CAD build for the part. Positions are in the model's coordinates, mm. Coordinates: 2 decimals unless noted, no trailing zeros. Loops run counter-clockwise (first coordinate to the right, second up) from the corner with the lowest first, then second, coordinate; pieces in that order, holes last. Notation, with made-up numbers: (1, -5) - (30, -5) arc R26 cw to (30, 12) - close; hole circle Ø6 at (46.5, 52.25). An arc over 180 degrees is marked (long way). Put each result on its own line as item: value.
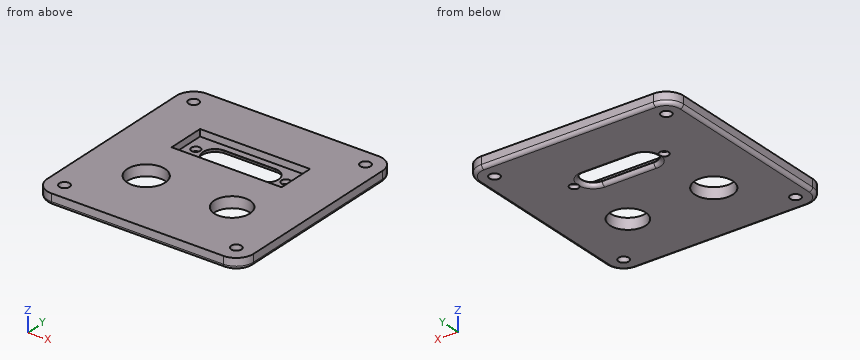
```python
from build123d import *

# Parameters (mm, degrees)
F0_W         = 76.2
F0_H         = 76.2
F0_R         = 1.905
F0_R_2       = 6.985
F0_R_3       = 6.604
F0_R_4       = 1.651
F1_DEPTH     = 1.524
F2_W         = 76.2
F2_H         = 76.2
F2_R         = 1.905
F2_W_2       = 40.64
F2_H_2       = 13.97
F3_DEPTH     = 2.54
F4_R         = 6.35
F5_T1_DEPTH  = 19.05
F5_T3_DEPTH  = 63.5
F5_T5_DEPTH  = 63.5
F5_T8_ANGLE  = 90
F5_T10_ANGLE = 90
F5_T12_ANGLE = 90
F5_T14_ANGLE = 90
F5_T16_ANGLE = 180
F5_T18_ANGLE = 180
F6_DEPTH     = 2.54


# Not quite as in the source:
# - a fillet or chamfer that OpenCascade refuses, or shapes differently, is made with other operations: its cross-section is extruded or revolved along the edge and cut away or added
# - a feature names something its author has since deleted; it is built from what else it names


with BuildPart() as f1:
    # F0 (on Top) → F1 (new body)
    with BuildSketch(Plane.XY):
        with Locations((0, -12.7)):
            Rectangle(F0_W, F0_H)
        with Locations((-31.75, -44.45)):
            Circle(F0_R, mode=Mode.SUBTRACT)
        with Locations((-15.875, -25.4)):
            Circle(F0_R_2, mode=Mode.SUBTRACT)
        with Locations((31.75, -44.45)):
            Circle(F0_R, mode=Mode.SUBTRACT)
        with Locations((15.875, -25.4)):
            Circle(F0_R_3, mode=Mode.SUBTRACT)
        with Locations((-16.637, 0)):
            Circle(F0_R_4, mode=Mode.SUBTRACT)
        with Locations((-31.75, 19.05)):
            Circle(F0_R, mode=Mode.SUBTRACT)
        with BuildLine():
            ThreePointArc((-9.525, -4.445), (-13.97, 0), (-9.525, 4.445))
            Line((-9.525, 4.445), (9.525, 4.445))
            ThreePointArc((9.525, 4.445), (13.97, 0), (9.525, -4.445))
            Line((9.525, -4.445), (-9.525, -4.445))
        make_face(mode=Mode.SUBTRACT)
        with Locations((16.637, 0)):
            Circle(F0_R_4, mode=Mode.SUBTRACT)
        with Locations((31.75, 19.05)):
            Circle(F0_R, mode=Mode.SUBTRACT)
    extrude(amount=F1_DEPTH)

    # F2 (on face) → F3 (join)
    with BuildSketch(Plane.XY.offset(1.524)):
        with Locations((0, -12.7)):
            Rectangle(F2_W, F2_H)
        with Locations((-31.75, -44.45)):
            Circle(F2_R, mode=Mode.SUBTRACT)
        with Locations((31.75, -44.45)):
            Circle(F2_R, mode=Mode.SUBTRACT)
        with Locations((-31.75, 19.05)):
            Circle(F2_R, mode=Mode.SUBTRACT)
        Rectangle(F2_W_2, F2_H_2, mode=Mode.SUBTRACT)
        with Locations((31.75, 19.05)):
            Circle(F2_R, mode=Mode.SUBTRACT)
    extrude(amount=F3_DEPTH)

    # F4
    f4_edges = [f1.edges().sort_by_distance(p)[0] for p in [
        (-38.1, -50.8, 2.032),
        (38.1, -50.8, 2.032),
        (-38.1, 25.4, 2.032),
        (38.1, 25.4, 2.032),
    ]]
    fillet(f4_edges, radius=F4_R)

    # F5: fillet of radius 1.27 on 12 edges, made by hand

    # F5_s2 → F5_t1 (cut)
    with BuildSketch(Plane.YZ.offset(-9.525)):
        with BuildLine():
            ThreePointArc((5.715, 0), (4.8169743879, 0.3719743879), (4.445, 1.27))
            Line((4.445, 1.27), (4.445, 0))
            Line((4.445, 0), (5.715, 0))
        make_face()
        with BuildLine():
            ThreePointArc((-5.715, 0), (-4.8169743879, 0.3719743879), (-4.445, 1.27))
            Line((-4.445, 1.27), (-4.445, 0))
            Line((-4.445, 0), (-5.715, 0))
        make_face()
    extrude(amount=F5_T1_DEPTH, mode=Mode.SUBTRACT)

    # F5_s4 → F5_t3 (cut)
    with BuildSketch(Plane.XZ.offset(-19.05)):
        with BuildLine():
            ThreePointArc((38.1, 1.27), (37.7280256121, 0.3719743879), (36.83, 0))
            Line((36.83, 0), (38.1, 0))
            Line((38.1, 0), (38.1, 1.27))
        make_face()
        with BuildLine():
            ThreePointArc((-36.83, 0), (-37.7280256121, 0.3719743879), (-38.1, 1.27))
            Line((-38.1, 1.27), (-38.1, 0))
            Line((-38.1, 0), (-36.83, 0))
        make_face()
    extrude(amount=F5_T3_DEPTH, mode=Mode.SUBTRACT)

    # F5_s6 → F5_t5 (cut)
    with BuildSketch(Plane.YZ.offset(-31.75)):
        with BuildLine():
            ThreePointArc((-49.53, 0), (-50.4280256121, 0.3719743879), (-50.8, 1.27))
            Line((-50.8, 1.27), (-50.8, 0))
            Line((-50.8, 0), (-49.53, 0))
        make_face()
        with BuildLine():
            ThreePointArc((24.13, 0), (25.0280256121, 0.3719743879), (25.4, 1.27))
            Line((25.4, 1.27), (25.4, 0))
            Line((25.4, 0), (24.13, 0))
        make_face()
    extrude(amount=F5_T5_DEPTH, mode=Mode.SUBTRACT)

    # F5_s7 → F5_t8 (revolve, cut)
    with BuildSketch(Plane.XZ.offset(44.45)):
        with BuildLine():
            ThreePointArc((-36.83, 0), (-37.7280256121, 0.3719743879), (-38.1, 1.27))
            Line((-38.1, 1.27), (-38.1, 0))
            Line((-38.1, 0), (-36.83, 0))
        make_face()
    revolve(axis=Axis((-31.75, -44.45, 0), (0, 0, 1)), revolution_arc=F5_T8_ANGLE, mode=Mode.SUBTRACT)

    # F5_s9 → F5_t10 (revolve, cut)
    with BuildSketch(Plane.XZ.offset(44.45)):
        with BuildLine():
            ThreePointArc((38.1, 1.27), (37.7280256121, 0.3719743879), (36.83, 0))
            Line((36.83, 0), (38.1, 0))
            Line((38.1, 0), (38.1, 1.27))
        make_face()
    revolve(axis=Axis((31.75, -44.45, 0), (0, 0, -1)), revolution_arc=F5_T10_ANGLE, mode=Mode.SUBTRACT)

    # F5_s11 → F5_t12 (revolve, cut)
    with BuildSketch(Plane.XZ.offset(-19.05)):
        with BuildLine():
            ThreePointArc((38.1, 1.27), (37.7280256121, 0.3719743879), (36.83, 0))
            Line((36.83, 0), (38.1, 0))
            Line((38.1, 0), (38.1, 1.27))
        make_face()
    revolve(axis=Axis((31.75, 19.05, 0), (0, 0, 1)), revolution_arc=F5_T12_ANGLE, mode=Mode.SUBTRACT)

    # F5_s13 → F5_t14 (revolve, cut)
    with BuildSketch(Plane.XZ.offset(-19.05)):
        with BuildLine():
            ThreePointArc((-36.83, 0), (-37.7280256121, 0.3719743879), (-38.1, 1.27))
            Line((-38.1, 1.27), (-38.1, 0))
            Line((-38.1, 0), (-36.83, 0))
        make_face()
    revolve(axis=Axis((-31.75, 19.05, 0), (0, 0, -1)), revolution_arc=F5_T14_ANGLE, mode=Mode.SUBTRACT)

    # F5_s15 → F5_t16 (revolve, cut)
    with BuildSketch(Plane.YZ.offset(-9.525)):
        with BuildLine():
            ThreePointArc((-5.715, 0), (-4.8169743879, 0.3719743879), (-4.445, 1.27))
            Line((-4.445, 1.27), (-4.445, 0))
            Line((-4.445, 0), (-5.715, 0))
        make_face()
    revolve(axis=Axis((-9.525, 0, 0), (0, 0, -1)), revolution_arc=F5_T16_ANGLE, mode=Mode.SUBTRACT)

    # F5_s17 → F5_t18 (revolve, cut)
    with BuildSketch(Plane.YZ.offset(9.525)):
        with BuildLine():
            ThreePointArc((5.715, 0), (4.8169743879, 0.3719743879), (4.445, 1.27))
            Line((4.445, 1.27), (4.445, 0))
            Line((4.445, 0), (5.715, 0))
        make_face()
    revolve(axis=Axis((9.525, 0, 0), (0, 0, -1)), revolution_arc=F5_T18_ANGLE, mode=Mode.SUBTRACT)

    # F6 (cut, through all): faces of the model
    f6_faces = [f1.faces().sort_by_distance(p)[0] for p in [
        (15.875, -25.4, 1.524),
        (-15.875, -25.4, 1.524),
    ]]
    extrude(f6_faces, amount=-F6_DEPTH, mode=Mode.SUBTRACT)


solid = f1.part
```
Q1. Pin check, flat tips, straight feed: pin 1 Ø4.5 at (x, y) = (16.637, 0) entering from -Z; pin 2 Ø5.5 at (x, y) = (-16.637, 0) entering from +Z. Stop position of each tip, or through.
Determined:
pin 1: z = 0
pin 2: z = 1.52
Q2. Wall check: L1, parallel to Y at x = 31.75, z = 1.75 (3 decimals); L2, parallel to Y at x = 32, z = 3.25; L3, parallel to Y at x = 6, z = 1.85 (3 decimals). Give the ranges that are in metal, low to high. Write a range as from..to.
Determined:
L1: -50.8..-46.355, -42.545..17.145, 20.955..25.4
L2: -50.8..-46.34, -42.56..17.16, 20.94..25.4
L3: -50.8..-6.985, 6.985..25.4
Q3. Slice it at A-A, the plane y = -25.4. Give the cut face in (x, z), then the cut area to 3 significant figures.
Determined:
outline: (-38.1, 1.27) arc R1.27 ccw to (-36.83, 0) - (-22.86, 0) - (-22.86, 4.06) - (-38.1, 4.06) - close; (-8.89, 0) - (9.27, 0) - (9.27, 4.06) - (-8.89, 4.06) - close; (22.48, 0) - (36.83, 0) arc R1.27 ccw to (38.1, 1.27) - (38.1, 4.06) - (22.48, 4.06) - close
area: 199 mm2
Q4. Slice it at B-B, the plane z = 3.35. Give the cut face in (x, y) (3 decimals).
Determined:
outline: (-38.1, -44.45) arc R6.35 ccw to (-31.75, -50.8) - (31.75, -50.8) arc R6.35 ccw to (38.1, -44.45) - (38.1, 19.05) arc R6.35 ccw to (31.75, 25.4) - (-31.75, 25.4) arc R6.35 ccw to (-38.1, 19.05) - close; hole circle Ø3.81 at (-31.75, -44.45); hole circle Ø3.81 at (-31.75, 19.05); hole circle Ø13.97 at (-15.875, -25.4); hole (-20.32, -6.985) - (20.32, -6.985) - (20.32, 6.985) - (-20.32, 6.985) - close; hole circle Ø13.208 at (15.875, -25.4); hole circle Ø3.81 at (31.75, -44.45); hole circle Ø3.81 at (31.75, 19.05)
